from build123d import *

# Parameters (mm, degrees)
ESQUISSE1_R        = 1.5
BOSS_EXTRU_1_DEPTH = 5


with BuildPart() as part:
    # Esquisse1 → Boss.-Extru.1 (new body)
    with BuildSketch(Plane(origin=(0, 0, 0), x_dir=(1, 0, 0), z_dir=(0, 1, 0))):
        Polygon((-58.927554829, 110), (-58.927554829, 160), (58.927554829, 160), (58.927554829, 110), (108.927554829, 110), (108.927554829, -110), (58.927554829, -110), (58.927554829, -160), (-58.927554829, -160), (-58.927554829, -110), (-108.927554829, -110), (-108.927554829, 0), (-108.927554829, 110), align=None)
        with Locations(Location((-103.976302336, -105, 0), (0, 0, 270))):
            Circle(ESQUISSE1_R, mode=Mode.SUBTRACT)
        with Locations(Location((-103.976302336, -55, 0), (0, 0, 270))):
            Circle(ESQUISSE1_R, mode=Mode.SUBTRACT)
        with Locations(Location((-53.976302336, -105, 0), (0, 0, 270))):
            Circle(ESQUISSE1_R, mode=Mode.SUBTRACT)
        with Locations(Location((-53.976302336, -155, 0), (0, 0, 270))):
            Circle(ESQUISSE1_R, mode=Mode.SUBTRACT)
        with Locations(Location((-53.976302336, 155, 0), (0, 0, 90))):
            Circle(ESQUISSE1_R, mode=Mode.SUBTRACT)
        with Locations(Location((-53.976302336, 105, 0), (0, 0, 90))):
            Circle(ESQUISSE1_R, mode=Mode.SUBTRACT)
        with Locations(Location((-103.976302336, 105, 0), (0, 0, 90))):
            Circle(ESQUISSE1_R, mode=Mode.SUBTRACT)
        with Locations(Location((-103.976302336, 55, 0), (0, 0, 90))):
            Circle(ESQUISSE1_R, mode=Mode.SUBTRACT)
        with Locations(Location((53.976302336, -155, 0), (0, 0, 90))):
            Circle(ESQUISSE1_R, mode=Mode.SUBTRACT)
        with Locations(Location((53.976302336, -105, 0), (0, 0, 90))):
            Circle(ESQUISSE1_R, mode=Mode.SUBTRACT)
        with Locations(Location((103.976302336, -105, 0), (0, 0, 90))):
            Circle(ESQUISSE1_R, mode=Mode.SUBTRACT)
        with Locations(Location((103.976302336, 105, 0), (0, 0, 270))):
            Circle(ESQUISSE1_R, mode=Mode.SUBTRACT)
        with Locations(Location((53.976302336, 105, 0), (0, 0, 270))):
            Circle(ESQUISSE1_R, mode=Mode.SUBTRACT)
        with Locations(Location((53.976302336, 155, 0), (0, 0, 270))):
            Circle(ESQUISSE1_R, mode=Mode.SUBTRACT)
    extrude(amount=BOSS_EXTRU_1_DEPTH)


solid = part.part
Verification items for the finished model (mm, model axes). Round coordinates to 2 decimals unless told otherwise and drop trailing zeros. Loops run counter-clockwise (first coordinate to the right, second up) from the corner with the lowest first, then second, coordinate; pieces in that order, holes last. Notation, with made-up numbers: (-11, 63.5) - (26, 63.5) arc R23 ccw to (26, 75.5) - close; hole circle Ø10 at (-23, 65.5). An arc over 180 degrees is marked (long way). Use a Markdown table: item, result. Add a question column.
1. Gauge pin test, flat end, axial feed: pin 1 (2.5 mm diameter, centred on y = 2, z = 134.5, fed in from -X). Record the tip position at first contact, or that the pin passes through.
2. Section check A-A, the plane y = 1.3. Give the number of separate pieces and of enclosed holes in the cut face, plus the area to 3 significant figures.
3. Section check B-B, the plane x = -87.5. Record the boundary of the cut face in (y, z), plus the area to 3 significant figures.
4. Thickness scan on probe 1 along X at (y, z) = (3.2, 155); probe 2 along Z at (x, y) = (-53.5, 4.5); probe 3 along X at (y, z) = (2, 105). Record the ranges inside material, lowest first. Write a range as [from, to].
Checks:
| question | item | result |
|---|---|---|
| 1 | pin 1 | stops at x = -58.93 |
| 2 | separate pieces | 1 |
| 2 | enclosed holes | 14 |
| 2 | area | 59,600 mm^2 |
| 3 | outline | (0, -110) - (5, -110) - (5, 110) - (0, 110) - close |
| 3 | area | 1,100 mm^2 |
| 4 | probe 1 | x = [-58.93, -55.48], [-52.48, 52.48], [55.48, 58.93] |
| 4 | probe 2 | z = [-160, -156.42], [-153.58, -106.42], [-103.58, 103.58], [106.42, 153.58], [156.42, 160] |
| 4 | probe 3 | x = [-108.93, -105.48], [-102.48, -55.48], [-52.48, 52.48], [55.48, 102.48], [105.48, 108.93] |
